Geometry: final body of the model. Coordinates: model frame, mm. A direction names the side the tool comes from. Give positions to 0.01 mm unless a question says otherwise; leave off trailing zeros. Loops run counter-clockwise (first coordinate to the right, second up) from the corner with the lowest first, then second, coordinate; pieces in that order, holes last. Notation, with made-up numbers: (30, -25.5) -> (68, -25.5) arc R33 ccw to (68, 10.5) -> close; hole circle Ø8 at (67, -21.5). An arc over 180 degrees is marked (long way). Answer in a Markdown table with one row per item. Add a question column.
1) Draft query along X for faces 1 (the conical face through (-35.816, 68.86, 41.868)), 2 (the conical face through (-43.1, 82.9, 16.4)), 3 (the flat face through (-25, 25, 0)). Return one class per face: +X half, -X half, draft (parallel to the pull), parting line (faces both ways), or undercut.
2) Section query D-D (z = 36.5). Return the cut outline in (x, y), plus the area to 3 significant figures.
3) Access query for faces 4 (the conical face through (-83.395, -26.262, 22.334)), 5 (the conical face through (80.921, 62.048, 17.514)). Directions: +Z, -Z, +X, -X, +Y, -Y. A direction counts if a zero-diameter tool reaches every point of the face in a straight line with its end or side. Return the directions, or none.
4) Section query C-C (z = 62.5). Return the cut outline in (x, y), plus the area to 3 significant figures.
5) Line query: line 1 (X direction, y = -9.5, z = 52.5); line 2 (Y direction, x = 15.5, z = 27); line 3 (X direction, y = 0, z = 43). Output: solid intervals per line, ascending. Write a range as from..to.
6) First-contact query: P1, Ø2, axis at x = 9.5, z = 14, coming from the -Y side; P2, Ø3, axis at y = 35.5, z = 40.5, coming from the -X side; P3, Ø5, axis at x = 48, z = 9.5, coming from the +Y side. Flat tips, straight axial feed; report the tip coordinate or a pass-through.
```python
from build123d import *

# Parameters (mm, degrees)
F2_R = 10


with BuildPart() as f1:
    # F0 (on Front) → F1 (revolve)
    with BuildSketch(Plane.XZ):
        with BuildLine():
            Line((-119.4852813742, 0), (-30, 0))
            Line((-30, 0), (-30, 75))
            ThreePointArc((-30, 75), (-33.7038994058, 80.5432771951), (-40.2426406871, 79.2426406871))
            Line((-40.2426406871, 79.2426406871), (-119.4852813742, 0))
        make_face()
    revolve(axis=Axis((0, 0, 44.6021817625), (0, 0, 1)))

    # F2 (on Front) → F3 (revolve, cut)
    with BuildSketch(Plane.XZ):
        with Locations((-70, 50)):
            Circle(F2_R)
    revolve(axis=Axis((0, 0, 44.2256368697), (0, 0, 1)), mode=Mode.SUBTRACT)

    # F4 (on Front) → F5 (revolve, cut)
    with BuildSketch(Plane.XZ):
        Polygon((-93.070267659, 16.2951581671), (-87.3115113074, 21.84824067), (-89.2412436485, 29.6120112161), (-96.929732341, 31.8226992593), (-102.6884886926, 26.2696167564), (-100.7587563515, 18.5058462103), align=None)
    revolve(axis=Axis((0, 0, 44.7207018733), (0, 0, 1)), mode=Mode.SUBTRACT)

    # F6 (on Front) → F7 (revolve, cut)
    with BuildSketch(Plane.XZ):
        Polygon((-50.2399520095, 78.2016961205), (-50.6398090678, 69.5098518968), (-41.9479648441, 69.1099948385), align=None)
    revolve(axis=Axis((0, 0, 44.9002496898), (0, 0, 1)), mode=Mode.SUBTRACT)


solid = f1.part
```
Evaluation:
| question | item | result |
|---|---|---|
| 1 | face 1 | parting line |
| 1 | face 2 | undercut |
| 1 | face 3 | draft |
| 2 | outline | circle Ø165.97 at (0, 0); hole circle Ø60 at (0, 0) |
| 2 | area | 18,800 mm² |
| 3 | face 4 | none |
| 3 | face 5 | +Z |
| 4 | outline | circle Ø113.97 at (0, 0); hole circle Ø60 at (0, 0) |
| 4 | area | 7,370 mm² |
| 5 | line 1 | -59.56..-28.46, 28.46..59.56 |
| 5 | line 2 | -87.23..-25.69, 25.69..87.23 |
| 5 | line 3 | -62.86..-30, 30..62.86 |
| 6 | P1 | y = -106.06 |
| 6 | P2 | x = -72.39 |
| 6 | P3 | y = 101.97 |
